Answer from the drawing. Dimensions are ordinates in mm from the lowest x, y and z of the part. A direction names the side the tool comes from. Coordinates: 2 decimals unless noted, no trailing zeros. Loops run counter-clockwise (first coordinate to the right, second up) from the corner with the lowest first, then second, coordinate; pieces in that order, holes last. Notation, with made-up numbers: (54.25, 51) -> (82.25, 51) arc R12 cw to (82.25, 64) -> close; hole circle Ø7 at (53.5, 57.25). An arc over 180 degrees is marked (long way). Use a Markdown table: item, result.
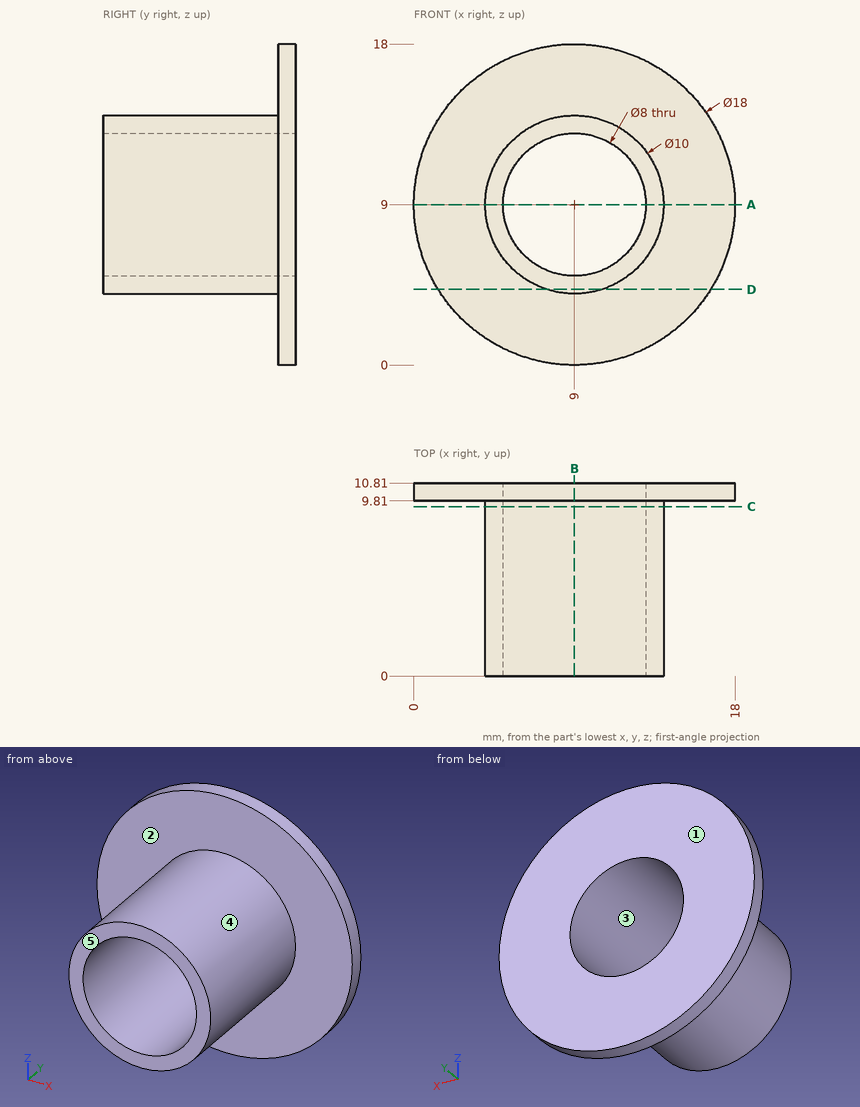
Q1. For the marked faces 1 and 2, determine the directions among +Z, -Z, +X, -X, +Y, -Y from which every point of the face is accessible in a straight line to the end or side of a thin tool.
Solved:
| item | result |
|---|---|
| face 1 | +Z, -Z, +X, -X, +Y |
| face 2 | -Y |
Q2. Section C-C on y = 9.5 is taken. Determine the outline of the cut face in (x, z), and give its area (3 significant figures).
Solved:
| item | result |
|---|---|
| outline | circle Ø10 at (9, 9); hole circle Ø8 at (9, 9) |
| area | 28.3 mm² |
Q3. Section A-A on z = 9 is taken. Determine the outline of the cut face in (x, y).
Solved:
| item | result |
|---|---|
| outline | (0, 9.81) -> (4, 9.81) -> (4, 0) -> (5, 0) -> (5, 10.81) -> (0, 10.81) -> close; (13, 0) -> (14, 0) -> (14, 9.81) -> (18, 9.81) -> (18, 10.81) -> (13, 10.81) -> close |
Q4. Section B-B on x = 9 is taken. Determine the outline of the cut face in (y, z).
Solved:
| item | result |
|---|---|
| outline | (0, 4) -> (9.81, 4) -> (9.81, 0) -> (10.81, 0) -> (10.81, 5) -> (0, 5) -> close; (0, 13) -> (10.81, 13) -> (10.81, 18) -> (9.81, 18) -> (9.81, 14) -> (0, 14) -> close |
Q5. Consider line 1 (Z direction, x = 9, y = 3); line 2 (Y direction, x = 13, z = 1.75). Determine where each line is inside the solid, lowest interval first. Write a range as [from, to].
Solved:
| item | result |
|---|---|
| line 1 | [4, 5], [13, 14] |
| line 2 | [9.81, 10.81] |
Q6. Determine the mould class of the marked faces 3, 4 and 5 for opening direction Z: pulls with the +Z half, pulls with the -Z half, needs draft (parallel to the pull), parting line crosses it, or undercut.
Solved:
| item | result |
|---|---|
| face 3 | undercut |
| face 4 | parting line crosses it |
| face 5 | needs draft |
Q7. Given pin 1 Ø5 at (y, z) = (4.5, 8) entering from +X; pin 2 Ø5 at (x, y) = (3, 5) entering from -Z, each flat-ended and moving along its own axis, determine where each tip first touches the part or whether it passes through.
Solved:
| item | result |
|---|---|
| pin 1 | x = 14 |
| pin 2 | z = 5.43 |
Q8. Section D-D on z = 4.25 is taken. Determine the outline of the cut face in (x, y), and give its area (3 significant figures).
Solved:
| item | result |
|---|---|
| outline | (1.36, 9.81) -> (7.44, 9.81) -> (7.44, 0) -> (10.56, 0) -> (10.56, 9.81) -> (16.64, 9.81) -> (16.64, 10.81) -> (1.36, 10.81) -> close |
| area | 45.9 mm² |
